```python
from build123d import *

# Parameters (mm, degrees)
PAD_DEPTH       = 10
SKETCH001_R     = 1.644392
SKETCH001_R_2   = 1.65157
SKETCH001_R_3   = 1.649148
SKETCH001_R_4   = 1.651214
SKETCH001_R_5   = 1.647788
SKETCH001_R_6   = 1.648804
SKETCH001_R_7   = 1.649175
SKETCH001_R_8   = 1.65022
POCKET_DEPTH    = 1177.994185
SKETCH002_R     = 1.5
POCKET001_DEPTH = 10.001


with BuildPart() as part:
    # Sketch → Pad (new body)
    with BuildSketch(Plane.XY):
        with BuildLine():
            ThreePointArc((-150.791263, -199.4041), (0, -250), (150.791263, -199.4041))
            Line((150.791263, 199.4041), (150.791263, -199.4041))
            ThreePointArc((150.791263, 199.4041), (0, 250), (-150.791263, 199.4041))
            Line((-150.791263, -199.4041), (-150.791263, 199.4041))
        make_face()
    extrude(amount=PAD_DEPTH)

    # Sketch001 (on Face6 of Pad) → Pocket (cut, through all)
    with BuildSketch(Plane.XY.offset(10)):
        with Locations((143.17194, 103.497585)):
            Circle(SKETCH001_R)
        with Locations((133.171706, 103.496141)):
            Circle(SKETCH001_R_2)
        with Locations((123.167499, 103.498465)):
            Circle(SKETCH001_R_3)
        with Locations((113.171268, 103.495805)):
            Circle(SKETCH001_R_4)
        with Locations((142.928472, 72.260962)):
            Circle(SKETCH001_R_5)
        with Locations((132.931272, 72.262033)):
            Circle(SKETCH001_R_6)
        with Locations((122.929515, 72.438862)):
            Circle(SKETCH001_R_7)
        with Locations((112.924957, 72.496527)):
            Circle(SKETCH001_R_8)
    pocket = extrude(amount=-POCKET_DEPTH, mode=Mode.SUBTRACT)

    # Mirrored: Pocket across Sketch001 V_Axis
    add(pocket.mirror(Plane(origin=(0, 0, 10), x_dir=(0, 0, 1), z_dir=(1, 0, 0))), mode=Mode.SUBTRACT)

    # Sketch002 (on DatumPlane) → Pocket001 (cut, through all)
    with BuildSketch(Plane.XY.offset(10)):
        with Locations((-19.594686, -202.247013)):
            Circle(SKETCH002_R)
        with Locations((10.42839, -203.084781)):
            Circle(SKETCH002_R)
        with Locations((-18.916492, -178.267013)):
            Circle(SKETCH002_R)
        with Locations((11.087714, -179.124447)):
            Circle(SKETCH002_R)
    extrude(amount=-POCKET001_DEPTH, mode=Mode.SUBTRACT)


solid = part.part
```
Input: part model. Units: mm. Frame: model coordinates. Give positions to 0.01 mm unless a question says otherwise; leave off trailing zeros. Write each loop counter-clockwise with the first axis right and the second up, starting at its lowest first coordinate (ties: lowest second). Pieces come first, ordered by that corner, then holes. Notation, with made-up numbers: (39, 83) - (60, 83) arc R8 cw to (60, 93) - close; hole circle Ø7 at (-32.75, 36.5). An arc over 180 degrees is marked (long way). Write item = value, one per line. Start each with the question number.
1. Section query B-B, the plane x = 58. Output: boundary loops of the cut face in (y, z).
2. Section query C-C, the plane x = -88.5. Output: boundary loops of the cut face in (y, z).
3. Section query A-A, the plane z = 6.75. Count the separate pieces of the cut face and the enclosed holes in it, then the cut area to 3 significant figures.
4. Mould query, pull axis Z, two halves, no side actions, for faces 1 (the flat face through (-2, 3, 0)), 2 (the cylindrical face through (2.27, 249.99, 4.93)), 3 (the flat face through (-2, 3, 10)). Classes: released by +Z, released by -Z, zero draft, split by the parting line, or undercut.
5. Ray query, L1, parallel to X at y = -202, z = 7.25; L2, parallel to Y at x = -122, z = 6.75; L3, parallel to Y at x = -112, z = 7.25. Return the intervals inside material, ascending.
6. First-contact query: pin 1 Ø1.5 at (x, z) = (-44, 6) entering from -Y; pin 2 Ø2 at (x, y) = (-122.93, 72.44) entering from -Z; pin 3 Ø6 at (x, z) = (-109, 7) entering from +Y; pin 4 Ø6 at (x, z) = (-76, 9) entering from +Y. Flat tips, straight axial feed; report the tip coordinate or a pass-through.
Check sheet entries:
q1.outline = (-243.18, 0) - (243.18, 0) - (243.18, 10) - (-243.18, 10) - close
q2.outline = (-233.81, 0) - (233.81, 0) - (233.81, 10) - (-233.81, 10) - close
q3.separate_pieces = 1
q3.enclosed_holes = 20
q3.area = 141,000 mm2
q4.face_1 = released by -Z
q4.face_2 = zero draft
q4.face_3 = released by +Z
q5.L1 = -147.3 to -21.07, -18.12 to 9.39, 11.46 to 147.3
q5.L2 = -218.21 to 71.08, 73.8 to 102.33, 104.66 to 218.21
q5.L3 = -223.51 to 71.13, 73.86 to 102.33, 104.66 to 223.51
q6.pin_1 = -246.23
q6.pin_2 = through
q6.pin_3 = 226.42
q6.pin_4 = 239.1
